```python
from build123d import *

# Parameters (mm, degrees)
F0_R     = 2.54
F1_DEPTH = 3.175


with BuildPart() as f1:
    # F0 (on Right) → F1 (new body)
    with BuildSketch(Plane.YZ):
        Polygon((2.176032, -36.759793), (2.176032, 80.715207), (-10.523968, 80.715207), (-10.523968, -29.427444), align=None)
        with Locations((-4.173968, 7.690207)):
            Circle(F0_R, mode=Mode.SUBTRACT)
        with Locations((-4.173968, 45.790207)):
            Circle(F0_R, mode=Mode.SUBTRACT)
    extrude(amount=F1_DEPTH)


solid = f1.part
```
Source: CAD feature listing. Evaluate the final solid. Frame: model axes, mm. Give positions to 0.01 mm unless a question says otherwise; leave off trailing zeros. Order: outer loops, then holes, each group sorted by start corner. A loop starts at its lowest first (then second) coordinate and runs counter-clockwise, first axis right, second up. Notation, with made-up numbers: (-7.75, 1.25) -> (43.25, 1.25) arc R32 ccw to (43.25, 39.25) -> close; hole circle Ø1 at (-25, 36). An arc over 180 degrees is marked (long way). Use a Markdown table: item, result.
Q1. Section B-B (y = -8.25). Return the cut outline in (x, z) (3 decimals).
A:
| item | result |
|---|---|
| outline | (0, -30.74) -> (3.175, -30.74) -> (3.175, 80.715) -> (0, 80.715) -> close |
Q2. First-contact query: P1, Ø3, axis at y = -4.17, z = 7.69, coming from the -X side. Flat tip, straight axial feed; report the tip coordinate or a pass-through.
A:
| item | result |
|---|---|
| P1 | through |
Q3. Section A-A (x = 1.25). Return the cut outline in (y, z).
A:
| item | result |
|---|---|
| outline | (-10.52, -29.43) -> (2.18, -36.76) -> (2.18, 80.72) -> (-10.52, 80.72) -> close; hole circle Ø5.08 at (-4.17, 7.69); hole circle Ø5.08 at (-4.17, 45.79) |
Q4. Material intervals for line 1 (Z direction, x = 2.7, y = -6.25); line 2 (Z direction, x = 2.15, y = -4.5); line 3 (Y direction, x = 1.7, z = 5.5), sorted ascending. Write a range as [from, to].
A:
| item | result |
|---|---|
| line 1 | [-31.9, 6.23], [9.15, 44.33], [47.25, 80.72] |
| line 2 | [-32.91, 5.17], [10.21, 43.27], [48.31, 80.72] |
| line 3 | [-10.52, -5.46], [-2.89, 2.18] |
Q5. Pull-direction query (Z, two-part tool) for faces 1 (the face through (3.175, -4, 23)), 2 (the face through (2, -4, 80.715)), 3 (the face through (1.57, -4.72, 43.31)); classes: +Z half, -Z half, draft (parallel to the pull), parting line (faces both ways), or undercut.
A:
| item | result |
|---|---|
| face 1 | draft |
| face 2 | +Z half |
| face 3 | undercut |
